The listing builds one solid part. Answer for the finished solid, in the listing's coordinates (mm). Face numbers are marked on the shaded views. Give positions to 0.01 mm unless a question says otherwise; leave off trailing zeros. Write each loop counter-clockwise with the first axis right and the second up, starting at its lowest first coordinate (ties: lowest second). Pieces come first, ordered by that corner, then holes. Notation, with made-up numbers: (42.5, 34) - (83.5, 34) arc R28 ccw to (83.5, 73) - close; hole circle Ø10 at (-16.75, 21). An arc over 180 degrees is marked (long way). Answer in a Markdown table with one row per item. Add a question column.
from build123d import *

# Parameters (mm, degrees)
SKETCH1_R           = 7.5
SKETCH1_R_2         = 5
BOSS_EXTRUDE1_DEPTH = 5
SKETCH2_R           = 7
SKETCH2_R_2         = 5.5
CUT_EXTRUDE1_DEPTH  = 0.5


with BuildPart() as part:
    # Sketch1 → Boss-Extrude1 (new body)
    with BuildSketch(Plane(origin=(0, 0, 0), x_dir=(1, 0, 0), z_dir=(0, 1, 0))):
        Circle(SKETCH1_R)
        Circle(SKETCH1_R_2, mode=Mode.SUBTRACT)
    extrude(amount=BOSS_EXTRUDE1_DEPTH)

    # Sketch2 → Cut-Extrude1 (cut)
    with BuildSketch(Plane(origin=(0, 5, 0), x_dir=(1, 0, 0), z_dir=(0, 1, 0))):
        Circle(SKETCH2_R)
        Circle(SKETCH2_R_2, mode=Mode.SUBTRACT)
    cut_extrude1 = extrude(amount=-CUT_EXTRUDE1_DEPTH, mode=Mode.SUBTRACT)

    # Mirror1: Cut-Extrude1 across plane
    add(cut_extrude1.mirror(Plane(origin=(0, 2.5, 0), x_dir=(0, 0, 1), z_dir=(0, -1, 0))), mode=Mode.SUBTRACT)


solid = part.part
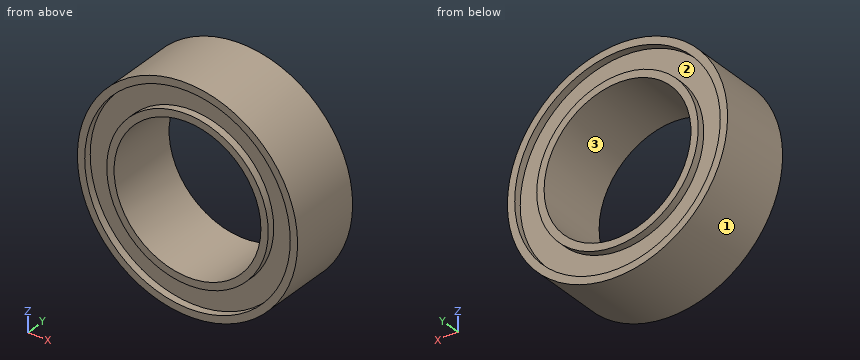
1. The mould has two halves that part along X. Classify the marked faces 1, 2 and 3: +X half, -X half, draft (parallel to the pull), parting line (faces both ways), or undercut.
2. Given pin 1 Ø6 at (x, z) = (0, 0) entering from -Y; pin 2 Ø1 at (x, y) = (5, 3) entering from +Z, each flat-ended and moving along its own axis, determine where each tip first touches the part or whether it passes through.
3. Section B-B (x = 0) is taken. Give the vertices of the cut face in (y, z).
4. Straight lines are drawn through the part: L1, parallel to Z at x = 0, y = 4.8; L2, parallel to X at y = 2.2, z = 0. For each, find the intervals that lie inside material, in ascending order. Write a range as [from, to].
5. Section A-A (z = 0) is taken. Give the vertices of the cut face in (x, y), and give its area (3 significant figures).
6. Section C-C (y = 3.7) is taken. Give the vertices of the cut face in (x, z).
Geometry check:
| question | item | result |
|---|---|---|
| 1 | face 1 | parting line |
| 1 | face 2 | undercut |
| 1 | face 3 | undercut |
| 2 | pin 1 | through |
| 2 | pin 2 | z = 6 |
| 3 | outline | (0, -7.5) - (5, -7.5) - (5, -7) - (4.5, -7) - (4.5, -5.5) - (5, -5.5) - (5, -5) - (0, -5) - (0, -5.5) - (0.5, -5.5) - (0.5, -7) - (0, -7) - close; (0, 5) - (5, 5) - (5, 5.5) - (4.5, 5.5) - (4.5, 7) - (5, 7) - (5, 7.5) - (0, 7.5) - (0, 7) - (0.5, 7) - (0.5, 5.5) - (0, 5.5) - close |
| 4 | L1 | [-7.5, -7], [-5.5, -5], [5, 5.5], [7, 7.5] |
| 4 | L2 | [-7.5, -5], [5, 7.5] |
| 5 | outline | (-7.5, 0) - (-7, 0) - (-7, 0.5) - (-5.5, 0.5) - (-5.5, 0) - (-5, 0) - (-5, 5) - (-5.5, 5) - (-5.5, 4.5) - (-7, 4.5) - (-7, 5) - (-7.5, 5) - close; (5, 0) - (5.5, 0) - (5.5, 0.5) - (7, 0.5) - (7, 0) - (7.5, 0) - (7.5, 5) - (7, 5) - (7, 4.5) - (5.5, 4.5) - (5.5, 5) - (5, 5) - close |
| 5 | area | 22.0 mm² |
| 6 | outline | circle Ø15 at (0, 0); hole circle Ø10 at (0, 0) |
